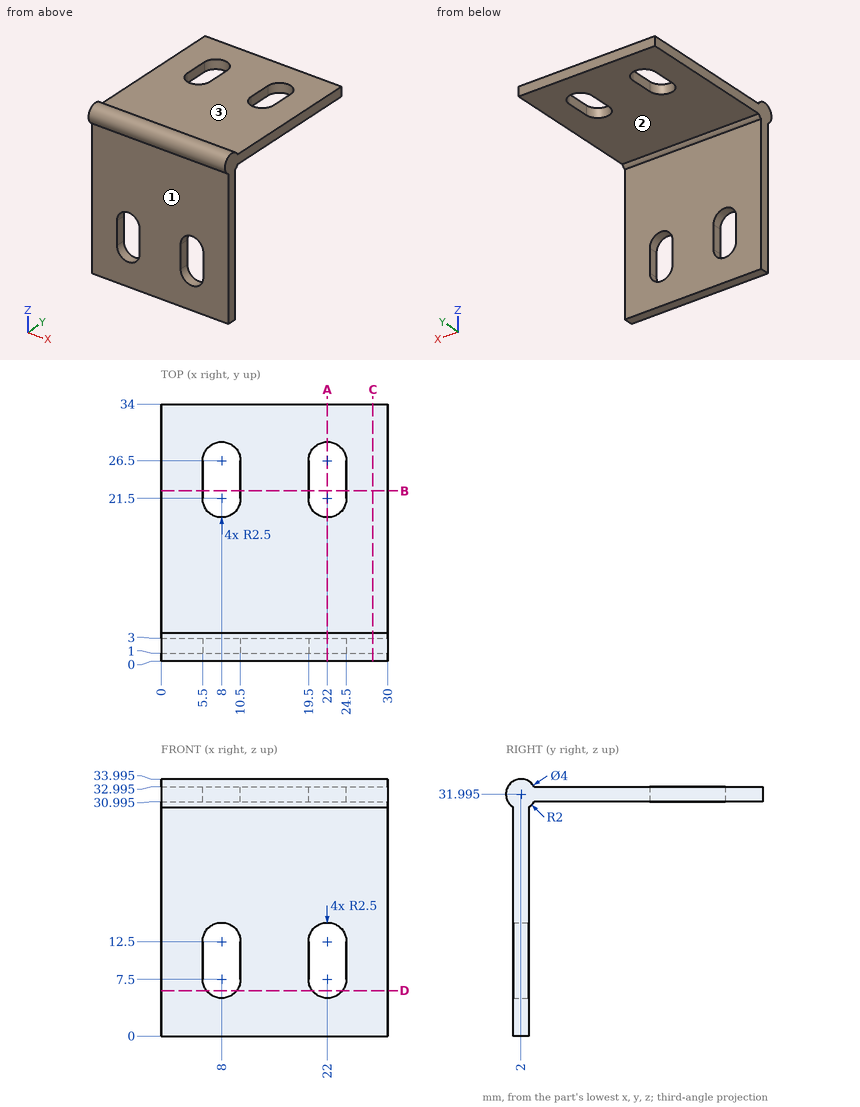
Drawing for the job (mm, zero at the part's lowest x, y, z). A direction names the side the tool comes from. Round coordinates to 2 decimals unless told otherwise and drop trailing zeros. Loops run counter-clockwise (first coordinate to the right, second up) from the corner with the lowest first, then second, coordinate; pieces in that order, holes last. Notation, with made-up numbers: (48, 84.25) - (88, 84.25) arc R32 ccw to (88, 111.25) - close; hole circle Ø4 at (-12.5, 76.5). An arc over 180 degrees is marked (long way). Return JSON: item names as keys, results as strings. Group by question number.
Q1. Band-saw the part on B-B on y = 22.5. Give the cut face in (x, z) (1 decimal), plus the area to 3 significant figures.
Q2. Drill centre lines: line 1 along Y through (x, z) = (5.75, 21); line 2 along Z through (x, y) = (3.25, 5) (1 decimal); line 3 along Z through (x, y) = (27.25, 3.5). Where is each one in solid material? Low to high. Write a range as [from, to].
Q3. Band-saw the part on C-C on x = 28. Give the cut face in (y, z) (1 decimal), plus the area to 3 significant figures.
Q4. Band-saw the part on A-A on x = 22. Give the cut face in (y, z) (1 decimal).
Q5. Band-saw the part on D-D on z = 6. Give the cut face in (x, y).
Q6. Tool access for the marked faces 1, 2 and 3: list every direction of +Z, -Z, +X, -X, +Y, -Y with a clear straight run to the whole face (end or side of a thin tool).
Q7. Flat gauge pins, fed straight in: pin 1 Ø15 at (x, y) = (18, 23) entering from -Z (3 decimals); pin 2 Ø9 at (x, y) = (18.5, 24) entering from +Z (3 decimals); pin 3 Ø15 at (x, z) = (21, 19.5) entering from +Y. Where does each tip first touch, or does it go through?
Solutions:
{
 "1": {"outline": "(0, 31) - (5.5, 31) - (5.5, 33) - (0, 33) - close; (10.5, 31) - (19.5, 31) - (19.5, 33) - (10.5, 33) - close; (24.5, 31) - (30, 31) - (30, 33) - (24.5, 33) - close", "area": "40.0 mm^2"},
 "2": {"line 1": "y = [1, 3]", "line 2": "z = [31, 33]", "line 3": "z = [30.67, 33.32]"},
 "3": {"outline": "(1, 0) - (3, 0) - (3, 30.3) arc R2 ccw to (3.7, 31) - (34, 31) - (34, 33) - (3.7, 33) arc R2 ccw (long way) to (1, 30.3) - close", "area": "133 mm^2"},
 "4": {"outline": "(1, 0) - (3, 0) - (3, 5) - (1, 5) - close; (1, 15) - (3, 15) - (3, 30.3) arc R2 ccw to (3.7, 31) - (19, 31) - (19, 33) - (3.7, 33) arc R2 ccw (long way) to (1, 30.3) - close; (29, 31) - (34, 31) - (34, 33) - (29, 33) - close"},
 "5": {"outline": "(0, 1) - (6, 1) - (6, 3) - (0, 3) - close; (10, 1) - (20, 1) - (20, 3) - (10, 3) - close; (24, 1) - (30, 1) - (30, 3) - (24, 3) - close"},
 "6": {"face 1": "-Z, +X, -X, -Y", "face 2": "-Z, +X, -X, +Y", "face 3": "+Z, +X, -X, +Y"},
 "7": {"pin 1": "stops at z = 30.995", "pin 2": "stops at z = 32.995", "pin 3": "stops at y = 3"}
}
